Autodesk Inventor part; units mm, degrees
ref_plane "YZ Plane" through (0, 0, 0) normal (1, 0, 0) x (0, 1, 0)
ref_plane "XZ Plane" through (0, 0, 0) normal (0, 1, 0) x (-1, 0, 0)
ref_plane "XY Plane" through (0, 0, 0) normal (0, 0, 1) x (1, 0, 0)
sketch "Sketch1" plane through (0, 0, 0) normal (0, 1, 0) x (-1, 0, 0)
  line L0 (7.5, -4.3301) -> (0, -8.6603)
  line L1 (0, -8.6603) -> (-7.5, -4.3301)
  line L2 (-7.5, -4.3301) -> (-7.5, 4.3301)
  line L3 (-7.5, 4.3301) -> (0, 8.6603)
  line L4 (0, 8.6603) -> (7.5, 4.3301)
  line L5 (7.5, 4.3301) -> (7.5, -4.3301)
  line L6 (-7.5, 0) -> (7.5, 0)
  line L7 (0, 8.6603) -> (0, -8.6603)
  point P0 (0, 0)
  point P1 (0, 0)
  dimension "d0" = 15
extrude "Extrusion1" add sketch "Sketch1" against normal blind 6.5
sketch "Sketch2" plane through (0, 0, 0) normal (1, 0, 0) x (0, 1, 0)
  point P0 (0, 0)
sketch "Sketch6" plane through (0, 0, 0) normal (1, 0, 0) x (0, 1, 0)
  line L0 (0, 8.6603) -> (0, 4.3301)
  line L1 (0, 4.3301) -> (-6.5, 4.3301)
  line L2 (-6.5, 8.6603) -> (-6.5, 4.3301)
  line L3 (0, 8.6603) -> (-6.5, 8.6603)
  line L4 (0, 8.6603) -> (0, 7.6603)
  line L5 (-0.5774, 8.6603) -> (0, 8.6603)
  line L6 (-0.5774, 8.6603) -> (0, 7.6603)
  line L7 (-0.3756, 0) -> (-10.093, 0)
  point P0 (0, 0)
  dimension "d6" = 1
  dimension "d7" = 30
revolve "Revolution1" cut sketch "Sketch6" angle 360 about axis through (0, -0.3756, 0) along (0, -1, 0) contours L0 L6 L3
sketch "Sketch7" plane through (0, 0, 0) normal (0, 1, 0) x (1, 0, 0)
  arc A0 (-5.0999, 5.7158) -> (-7.5, 1.5587) centre (0, 0) ccw
hole "Hole1" at (0, 0, 0) direction (0, -1, 0) diameter 6.647 end through all
properties part number "M8_driving_nut"
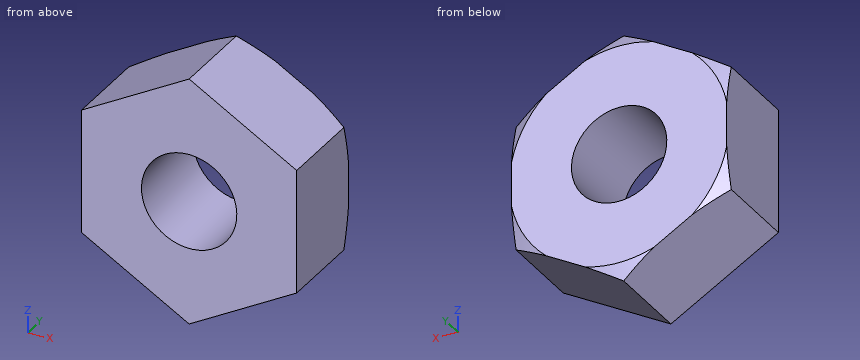
Model file for the job. Use its own axes, mm. Give positions to 0.01 mm unless a question says otherwise; leave off trailing zeros. Loops run counter-clockwise (first coordinate to the right, second up) from the corner with the lowest first, then second, coordinate; pieces in that order, holes last. Notation, with made-up numbers: (-14.75, 50) - (-5.75, 50) arc R15 ccw to (-5.75, 78) - close; hole circle Ø4 at (25.5, 63). An arc over 180 degrees is marked (long way). One line per item, written item: value. Start each with the question number.
1. Pin check, flat tips, straight feed: pin 1 (3 mm diameter, centred on x = -5.5, y = -2, fed in from +Z); pin 2 (2 mm diameter, centred on x = 3, y = -1.5, fed in from -Z). Stop position of each tip, or through.
2. Probe L1, parallel to X at y = -2.75, z = 0; L2, parallel to Z at x = 0, y = -0.5; L3, parallel to Z at x = -2.5, y = -1.75. List the from-to ranges inside material, lowest first. Write a range as from..to.
3. Slice it at A-A (z = 0). List the corners of the cut face in (x, y).
4. Slice it at C-C (z = 6.75). List the corners of the cut face in (x, y), plus the area to 3 significant figures.
5. Slice it at B-B (y = -4.5). List the corners of the cut face in (x, z), plus the area to 3 significant figures.
6. Slice it at D-D (x = 4.25). List the corners of the cut face in (y, z).
Solution:
1. pin 1: stops at z = 6.35
1. pin 2: stops at z = -7.51
2. L1: x = -7.5..-3.32, 3.32..7.5
2. L2: z = -8.53..-3.32, 3.32..8.53
2. L3: z = -7.22..-2.19, 2.19..7.22
3. outline: (-7.5, -6.5) - (-3.32, -6.5) - (-3.32, 0) - (-7.5, 0) - close; (3.32, -6.5) - (7.5, -6.5) - (7.5, 0) - (3.32, 0) - close
4. outline: (-3.31, -6.5) - (3.31, -6.5) - (3.31, 0) - (-3.31, 0) - close
4. area: 43.0 mm^2
5. outline: (-7.5, -4.33) - (0, -8.66) - (7.5, -4.33) - (7.5, 4.33) - (0, 8.66) - (-7.5, 4.33) - close; hole circle Ø6.65 at (0, 0)
5. area: 160 mm^2
6. outline: (-6.5, -6.21) - (0, -6.21) - (0, 6.21) - (-6.5, 6.21) - close
